For this review, take the finished solid that the model builds, in its own axes (mm). Round coordinates to 2 decimals unless told otherwise and drop trailing zeros. Write each loop counter-clockwise with the first axis right and the second up, starting at its lowest first coordinate (ties: lowest second). Pieces come first, ordered by that corner, then holes.
from build123d import *

# Parameters (mm, degrees)
SKETCH1_R           = 1.5
SKETCH1_R_2         = 2.1
SKETCH1_R_3         = 2.175
BOSS_EXTRUDE3_DEPTH = 3


with BuildPart() as part:
    # Sketch1 → Boss-Extrude3 (new body)
    with BuildSketch(Plane.XY):
        with BuildLine():
            Line((-128.173606683, 10.293399025), (-76.045238805, 45.70647235))
            ThreePointArc((-76.045238805, 45.70647235), (-53.507275984, 56.931628533), (-28.795238805, 61.75647235))
            Line((-28.795238805, 61.75647235), (72.257182683, 67.642360637))
            Line((72.257182683, 67.642360637), (86.853615252, 71.437479344))
            ThreePointArc((86.853615252, 71.437479344), (91.314459888, 77.20647235), (86.853615252, 82.975465356))
            Line((86.853615252, 82.975465356), (75.443530199, 86.236617693))
            Line((75.443530199, 86.236617693), (72.32406126, 86.780586344))
            Line((72.32406126, 86.780586344), (-33.295238805, 93.85647235))
            ThreePointArc((-33.295238805, 93.85647235), (-46.44497492, 93.411826928), (-59.240002329, 90.345796421))
            ThreePointArc((-59.240002329, 90.345796421), (-71.070665181, 84.517465038), (-81.145238805, 76.00647235))
            Line((-81.145238805, 76.00647235), (-135.858404881, 19.427395317))
            ThreePointArc((-135.858404881, 19.427395317), (-136.13643621, 11.393713442), (-128.173606683, 10.293399025))
        make_face()
        with Locations((85.204761195, 77.20647235)):
            Circle(SKETCH1_R, mode=Mode.SUBTRACT)
        with Locations((-45.295238805, 73.911181311)):
            Circle(SKETCH1_R_2, mode=Mode.SUBTRACT)
        with Locations((-131.545238805, 15.25647235)):
            Circle(SKETCH1_R_3, mode=Mode.SUBTRACT)
        with Locations((-57.927136979, 73.911181311)):
            Circle(SKETCH1_R, mode=Mode.SUBTRACT)
        with Locations((-30.210957337, 78.946585736)):
            Circle(SKETCH1_R, mode=Mode.SUBTRACT)
    extrude(amount=BOSS_EXTRUDE3_DEPTH)


solid = part.part
(1) We need section C-C, the plane y = 31.5. Give the boundary of the cut face in (x, z).
Geometry check:
outline: (-124.18, 0) - (-96.96, 0) - (-96.96, 3) - (-124.18, 3) - close
(2) Mouldability with a two-part tool opening along X and no side actions: class faces 1 (the face through (-32, 68, 0)), 2 (the face through (-129.47, 15.91, 1.48)), 3 (the face through (-46.843, 75.33, 1.479)), 4 (the face through (-102.474, 27.752, 1.479)) as pulls with the +X half, pulls with the -X half, needs draft (parallel to the pull), parting line crosses it, or undercut.
Geometry check:
face 1: needs draft
face 2: undercut
face 3: undercut
face 4: pulls with the +X half
(3) For pin 1 Ø2.5 at (x, y) = (85.2, 77.21) entering from +Z; pin 2 Ø1.5 at (x, z) = (22, 1) entering from +Y; pin 3 Ø5 at (x, y) = (-131.55, 15.26) entering from +Z, all flat-tipped, find the tip position at first contact; note any pin that passes through.
Geometry check:
pin 1: passes through
pin 2: stops at y = 90.2
pin 3: stops at z = 3
(4) We need section B-B, the plane x = -3.5. Give the boundary of the cut face in (y, z), and give its area (3 significant figures).
Geometry check:
outline: (63.23, 0) - (91.86, 0) - (91.86, 3) - (63.23, 3) - close
area: 85.9 mm2
(5) For line 1 along X through (y, z) = (15.5, 1.9); line 2 along Y through (x, z) = (17.5, 2.55); line 3 along X through (y, z) = (80.5, 1.4), list the stretches that pass through material, from the lowest coordinate up.
Geometry check:
line 1: x = -137.54 to -133.71, -129.38 to -120.51
line 2: y = 64.45 to 90.45
line 3: x = -76.45 to 90.32
(6) We need section A-A, the plane z = 0.45. Give the boundary of the cut face in (x, y) (3 decimals), and give its area (3 significant figures).
Geometry check:
outline: (-135.858, 19.427) arc R6 ccw to (-128.174, 10.293) - (-76.045, 45.706) arc R93.789 cw to (-28.795, 61.756) - (72.257, 67.642) - (86.854, 71.437) arc R5.961 ccw to (86.854, 82.975) - (75.444, 86.237) - (72.324, 86.781) - (-33.295, 93.856) arc R65.442 ccw to (-59.24, 90.346) arc R54.247 ccw to (-81.145, 76.006) - close; hole circle Ø4.35 at (-131.545, 15.256); hole circle Ø3 at (-57.927, 73.911); hole circle Ø4.2 at (-45.295, 73.911); hole circle Ø3 at (-30.211, 78.947); hole circle Ø3 at (85.205, 77.206)
area: 5,910 mm2
